Geometry check sheet. Reference: drawing and pictorial views, mm from the part's lowest x, y, z. Give positions to 0.01 mm unless a question says otherwise; leave off trailing zeros. Order: outer loops, then holes, each group sorted by start corner. A loop starts at its lowest first (then second) coordinate and runs counter-clockwise, first axis right, second up. Notation, with made-up numbers: (36, 22.25) - (51, 22.25) arc R14 ccw to (51, 27.25) - close; hole circle Ø3 at (-30, 48.25). An arc over 180 degrees is marked (long way). Answer as a JSON object with one key per item and string values.
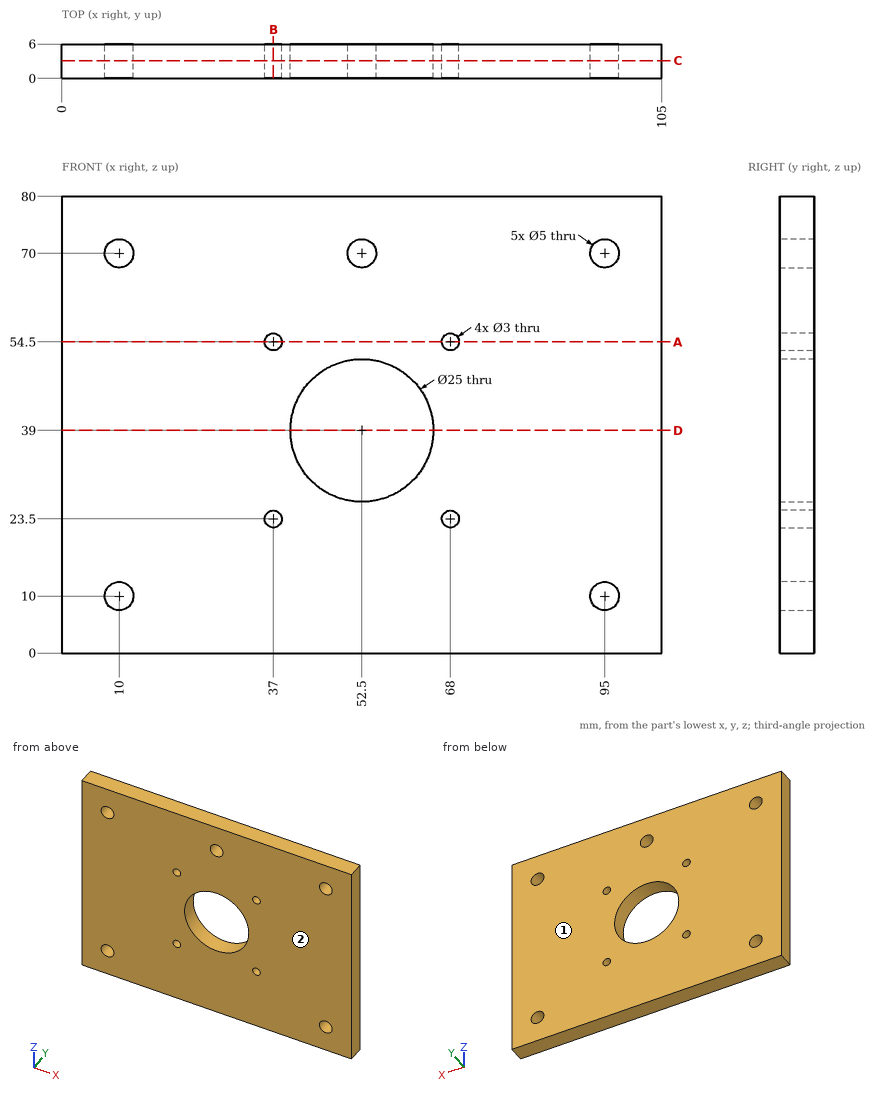
(1) Section check C-C (y = 3.1). Count the separate pieces of the cut face and the enclosed holes in it, then the cut area to 3 significant figures.
Computed values:
{"separate pieces": "1", "enclosed holes": "10", "area": "7,780 mm²"}
(2) Release check for a two-part mould opening along Y. For the marked faces 1 and 2 record: pulls with the +Y half, pulls with the -Y half, needs draft (parallel to the pull), parting line crosses it, or undercut.
Computed values:
{"face 1": "pulls with the +Y half", "face 2": "pulls with the -Y half"}
(3) Section check D-D (z = 39). Record the cut outline in (x, y), then the cut area to 3 significant figures.
Computed values:
{"outline": "(0, 0) - (40, 0) - (40, 6) - (0, 6) - close; (65, 0) - (105, 0) - (105, 6) - (65, 6) - close", "area": "480 mm²"}
(4) Section check B-B (x = 37). Record the cut outline in (y, z), then the cut area to 3 significant figures.
Computed values:
{"outline": "(0, 0) - (6, 0) - (6, 22) - (0, 22) - close; (0, 25) - (6, 25) - (6, 53) - (0, 53) - close; (0, 56) - (6, 56) - (6, 80) - (0, 80) - close", "area": "444 mm²"}
(5) Material ranges on line 1 along X through (y, z) = (2.2, 70); line 2 along X through (y, z) = (4.25, 23.5); line 3 along Z through (x, y) = (95, 1.75), recorded low to high. Write a range as [from, to].
Computed values:
{"line 1": "x = [0, 7.5], [12.5, 50], [55, 92.5], [97.5, 105]", "line 2": "x = [0, 35.5], [38.5, 66.5], [69.5, 105]", "line 3": "z = [0, 7.5], [12.5, 67.5], [72.5, 80]"}
(6) Section check A-A (z = 54.5). Record the cut outline in (x, y).
Computed values:
{"outline": "(0, 0) - (35.5, 0) - (35.5, 6) - (0, 6) - close; (38.5, 0) - (66.5, 0) - (66.5, 6) - (38.5, 6) - close; (69.5, 0) - (105, 0) - (105, 6) - (69.5, 6) - close"}
